from build123d import *

# Parameters (mm, degrees)
F1_DEPTH = 27.178


with BuildPart() as f1:
    # F0 (on Right) → F1 (new body)
    with BuildSketch(Plane.YZ):
        Polygon((-201.0527832023, 103.0996836883), (-111.1142710685, 75.0100706926), (-195.7207322121, 131.6622793674), align=None)
        Polygon((-111.1142710685, 75.0100706926), (-206.2715808406, 74.0581721357), (-206.0097499806, 73.8894074276), (0, 0), (210.9516762065, -77.6375151615), (-101.6242206097, 131.6622793674), align=None)
        Polygon((-206.4524721431, 74.174766749), (-206.2715808406, 74.0581721357), (-111.1142710685, 75.0100706926), (-201.0527832023, 103.0996836883), align=None)
        Polygon((-205.8051467933, 73.7575291716), (-206.4746171236, 74.0561410785), (-85.4999272821, -8.3092013374), (17.7439041436, -77.6375151615), (0, -25.8079376072), (-85.4999272821, -3.785947777), align=None)
        Polygon((-33.874746412, -2.9306560755), (-205.8051467933, 73.7575291716), (-85.4999272821, -3.785947777), (0, -2.9306560755), (0, -25.8079376072), (17.7439041436, -77.6375151615), (210.9516762065, -77.6375151615), (0, 0), align=None)
        Polygon((-292.5057113171, 131.6622793674), (-211.7819928518, 77.6099424455), (-206.4524721431, 74.174766749), (-201.0527832023, 103.0996836883), align=None)
        Polygon((-195.7207322121, 131.6622793674), (-292.5057113171, 131.6622793674), (-201.0527832023, 103.0996836883), align=None)
    extrude(amount=F1_DEPTH)


solid = f1.part
Work out the finished part from the listing and answer in its coordinate system (mm). A direction names the side the tool comes from. Give positions to 0.01 mm unless a question says otherwise; leave off trailing zeros. Loops run counter-clockwise (first coordinate to the right, second up) from the corner with the lowest first, then second, coordinate; pieces in that order, holes last. Notation, with made-up numbers: (2, 64.25) -> (10, 64.25) arc R28 ccw to (10, 84.25) -> close; hole circle Ø9 at (23, 51). An arc over 180 degrees is marked (long way). Use a Markdown table: item, result. Add a question column.
1. Flat-ended cylindrical pins translate along their axes: pin 1 Ø1 at (x, y) = (9, -240.5) entering from -Z; pin 2 Ø5 at (x, y) = (5, -137.5) entering from -Z; pin 3 Ø2 at (x, y) = (16, -69.5) entering from +Z. Find the tip coordinate at first contact, or state that the pin passes through.
2. Section B-B on z = 103 is taken. Determine the outline of the cut face in (x, y).
3. Determine the mould class of faces 4 (the flat face through (13, -243, 131.662)), 5 (the flat face through (13.399, -104.447, 37.462)), 6 (the flat face through (13.399, -146.834, 33.45)) for opening direction Y: released by +Y, released by -Y, zero draft, split by the parting line, or undercut.
4. Find the intervals of material crossed by probe 1 along Z at (x, y) = (19, -47); probe 2 along Z at (x, y) = (21.25, -42.5); probe 3 along Y at (x, z) = (5.75, 83.5), in increasing order.
5. Section C-C on y = -120 is taken. Determine the outline of the cut face in (x, z), and give its area (3 significant figures).
6. Section D-D on y = -64 is taken. Determine the outline of the cut face in (x, z).
7. Section A-A on x = 19.5 is taken. Determine the outline of the cut face in (y, z), and give its area (3 significant figures).
8. For faces 1 (the flat face through (13.399, -152.825, 102.94)), 2 (the flat face through (13, 0, -14)), 3 (the flat face through (13.4, -34.6, -42.49)), determine the directions among +Z, -Z, +X, -X, +Y, -Y from which every point of the face is accessible in a straight line to the end or side of a thin tool.
Results below:
| question | item | result |
|---|---|---|
| 1 | pin 1 | stops at z = 96.5 |
| 1 | pin 2 | stops at z = 25.39 |
| 1 | pin 3 | stops at z = 110.82 |
| 2 | outline | (0, -249.7) -> (27.18, -249.7) -> (27.18, -152.92) -> (0, -152.92) -> close; (0, -106.43) -> (27.18, -106.43) -> (27.18, -58.82) -> (0, -58.82) -> close |
| 3 | face 4 | zero draft |
| 3 | face 5 | undercut |
| 3 | face 6 | released by -Y |
| 4 | probe 1 | z = -34.16 to -13.7, -3.4 to 2.92, 16.86 to 95.09 |
| 4 | probe 2 | z = -37.18 to -14.86, -3.36 to 0.92, 15.24 to 92.07 |
| 4 | probe 3 | y = -220.58 to -123.79, -109.69 to -29.7 |
| 5 | outline | (0, 15.18) -> (27.18, 15.18) -> (27.18, 35.48) -> (0, 35.48) -> close; (0, 43.04) -> (27.18, 43.04) -> (27.18, 80.96) -> (0, 80.96) -> close |
| 5 | area | 1,580 mm^2 |
| 6 | outline | (0, -22.75) -> (27.18, -22.75) -> (27.18, -9.32) -> (0, -9.32) -> close; (0, -3.57) -> (27.18, -3.57) -> (27.18, 10.51) -> (0, 10.51) -> close; (0, 22.95) -> (27.18, 22.95) -> (27.18, 106.47) -> (0, 106.47) -> close |
| 7 | outline | (-292.51, 131.66) -> (-211.78, 77.61) -> (-206.01, 73.89) -> (0, 0) -> (-33.87, -2.93) -> (-206.47, 74.06) -> (-85.5, -8.31) -> (17.74, -77.64) -> (210.95, -77.64) -> (-101.62, 131.66) -> (-111.11, 75.01) -> (-195.72, 131.66) -> close; hole (-85.5, -3.79) -> (0, -25.81) -> (0, -2.93) -> close |
| 7 | area | 35,000 mm^2 |
| 8 | face 1 | +Z, +X, -X |
| 8 | face 2 | +X, -X |
| 8 | face 3 | -Z, +X, -X, -Y |
